Autodesk Inventor part; units mm, degrees
ref_plane "YZ Plane" through (0, 0, 0) normal (1, 0, 0) x (0, 1, 0)
ref_plane "XZ Plane" through (0, 0, 0) normal (0, 1, 0) x (-1, 0, 0)
ref_plane "XY Plane" through (0, 0, 0) normal (0, 0, 1) x (1, 0, 0)
sketch "Szkic1" plane through (0, 0, 0) normal (0, 0, 1) x (1, 0, 0)
  circle A0 centre (0, 0) radius 7
  dimension "d0" = 14
extrude "Wyciągnięcie proste1" add sketch "Szkic1" along normal blind 50
sketch "Szkic2" plane through (0, 0, 50) normal (0, 0, 1) x (1, 0, 0)
  circle A0 centre (0, 0) radius 2
  dimension "d3" = 4
extrude "Wyciągnięcie proste2" add sketch "Szkic2" along normal blind 1
fillet "Zaokrąglenie1" radius 0.25 2 edges at (-2, 0, 51) (-2, 0, 50)
fillet "Zaokrąglenie2" radius 1 2 edges at (-7, 0, 50) (-7, 0, 0)
properties part number "Bateria"
Can you work these out from the model? Positions are in its coordinate system, mm. A direction names the side the tool comes from. Coordinates: 2 decimals unless noted, no trailing zeros. Loops run counter-clockwise (first coordinate to the right, second up) from the corner with the lowest first, then second, coordinate; pieces in that order, holes last. Notation, with made-up numbers: (13.25, 30) -> (35.25, 30) arc R27 cw to (35.25, 49) -> close; hole circle Ø3 at (25.5, -0.75). An arc over 180 degrees is marked (long way). Answer as a JSON object with one key per item and string values.
1) For faces 1 (the face through (0, 0, 0)), 2 (the face through (-0.434, 1.952, 50.496)), which set-ups out of +Z, -Z, +X, -X, +Y, -Y let a thin tool reach every point of the face, with its end or its side?
Results:
{"face 1": "-Z, +X, -X, +Y, -Y", "face 2": "+Z"}
2) Imagine slicing it at A-A (y = 0). Please give me the cut outline in (x, z), then the cut area to 3 significant figures.
Results:
{"outline": "(-7, 1) arc R1 ccw to (-6, 0) -> (6, 0) arc R1 ccw to (7, 1) -> (7, 49) arc R1 ccw to (6, 50) -> (2.25, 50) arc R0.25 cw to (2, 50.25) -> (2, 50.75) arc R0.25 ccw to (1.75, 51) -> (-1.75, 51) arc R0.25 ccw to (-2, 50.75) -> (-2, 50.25) arc R0.25 cw to (-2.25, 50) -> (-6, 50) arc R1 ccw to (-7, 49) -> close", "area": "703 mm^2"}
3) If I drill on line 1 (Z direction, x = 3, y = 4.75); line 2 (X direction, y = 2.75, z = 28); line 3 (X direction, y = -5.5, z = 38.5), over which ranges is the centre line in solid material (lowest first)?
Results:
{"line 1": "z = 0 to 50", "line 2": "x = -6.44 to 6.44", "line 3": "x = -4.33 to 4.33"}
4) For P1, Ø1.5, axis at y = 2, z = 13.5, coming from the -X side; P2, Ø1.5, axis at y = 2.5, z = 8.5, coming from the -X side; P3, Ø2, axis at x = 1, z = 42.5, coming from the +Y side, each with a flat end and sliding along its axis, tell me the tip position at first contact or that it passes through.
Results:
{"P1": "stops at x = -6.89", "P2": "stops at x = -6.78", "P3": "stops at y = 7"}
5) Imagine slicing it at C-C (z = 13). Please give me the cut outline in (x, y), then the cut area to 3 significant figures.
Results:
{"outline": "circle Ø14 at (0, 0)", "area": "154 mm^2"}
